Read the model definition and answer for the solid it produces. Units are mm, in the model's axes. Face numbers are marked on the shaded views. A direction names the side the tool comes from. Coordinates: 2 decimals unless noted, no trailing zeros. Loops run counter-clockwise (first coordinate to the right, second up) from the corner with the lowest first, then second, coordinate; pieces in that order, holes last. Notation, with made-up numbers: (23.25, -1.75) -> (40.25, -1.75) arc R37 cw to (40.25, 37.25) -> close; hole circle Ø6 at (21.25, -16.75). An arc over 180 degrees is marked (long way). Answer as a JSON object with one key per item and string values. Group by question number.
Q1. The part is cut by section D-D on y = 0. State how many separate pieces and enclosed holes the cut face has, and give its area (3 significant figures).
Q2. Each of these flat-tipped pins is pushed along its axis until it touches: P1, Ø2.5, axis at x = -7.2, y = 0, coming from the +Z side; P2, Ø3.5, axis at x = 0, y = -7.2, coming from the -Z side; P3, Ø8, axis at x = -5, z = -9, coming from the -Y side; P4, Ø4.5, axis at x = -1, y = 1, coming from the -Z side. Where does it stop, or does it pass through?
Q3. Determine the mould class of the marked faces 1, 2 and 3 for opening direction X: released by +X, released by -X, zero draft, split by the parting line, or undercut.
Q4. Straight lines are drawn through the part: line 1 along Y through (x, z) = (0, -0.7) (3 decimals); line 2 along Z through (x, y) = (4.75, -0.75); line 3 along Z through (x, y) = (5.5, 4.75). For each, find the intervals that lie inside material, in ascending order. Write a range as [from, to].
Q5. The part is cut by section A-A on y = 7.2. Write down the section's boundary in (x, z) (3 decimals), and give its area (3 significant figures).
Q6. The part is cut by section B-B on z = -1.5. Write down the section's boundary in (x, y) (3 decimals).
Q7. For the marked faces 4 and 5, determine the directions among +Z, -Z, +X, -X, +Y, -Y from which every point of the face is accessible in a straight line to the end or side of a thin tool.
from build123d import *

# Parameters (mm, degrees)
SKETCH_1_R               = 5
EXTRUDE_1_DEPTH          = 19.4
SKETCH_2_R               = 9.3
EXTRUDE_2_DEPTH          = 2.5
EXTRUDE_START            = 14.1
SKETCH_3_R               = 5
EXTRUDE_3_DEPTH          = 14.1
SKETCH_5_W               = 0.3
SKETCH_5_H               = 1.1
SKETCH_6_W               = 0.3
SKETCH_6_H               = 1.1
HOLE_WIZARD_M2_5_2_D     = 2.05
HOLE_WIZARD_M2_5_2_DEPTH = 7.25
HOLE_WIZARD_M2_5_2_TIP   = 0.591784026
SKETCH_12_R              = 2
CUT_EXTRUDE_1_DEPTH      = 28


with BuildPart() as part:
    # 草图1 → 凸台-拉伸1 (new body)
    with BuildSketch(Plane.XY):
        Circle(SKETCH_1_R)
    extrude(amount=EXTRUDE_1_DEPTH)

    # 草图2 → 凸台-拉伸2 (add)
    with BuildSketch(Plane(origin=(0, 0, 0), x_dir=(-1, 0, 0), z_dir=(0, 0, -1))):
        Circle(SKETCH_2_R)
    extrude(amount=EXTRUDE_2_DEPTH)

    # 草图3 → 凸台-拉伸3 (add)
    with BuildSketch(Plane(origin=(0, 0, -2.5), x_dir=(-1, 0, 0), z_dir=(0, 0, -1)).offset(EXTRUDE_START)):
        with Locations(Location((0, 0, 0), (0, 0, 180))):
            Circle(SKETCH_3_R)
    extrude(amount=-EXTRUDE_3_DEPTH)

    # 草图5 → 切除-旋转3 (revolve, cut)
    with BuildSketch(Plane(origin=(0, 0, 0), x_dir=(1, 0, 0), z_dir=(0, 1, 0)), mode=Mode.PRIVATE) as cut_revolve_3_sk:
        with Locations((4.85, 14.15)):
            Rectangle(SKETCH_5_W, SKETCH_5_H)
    revolve(cut_revolve_3_sk.sketch.rotate(Axis((0, 0, -16.6), (0, 0, 1)), 180), axis=Axis((0, 0, -16.6), (0, 0, 1)), mode=Mode.SUBTRACT)

    # 草图6 → 切除-旋转4 (revolve, cut)
    with BuildSketch(Plane(origin=(0, 0, 0), x_dir=(1, 0, 0), z_dir=(0, 1, 0))):
        with Locations((4.85, -16.95)):
            Rectangle(SKETCH_6_W, SKETCH_6_H)
    revolve(axis=Axis((0, 0, 19.4), (0, 0, -1)), mode=Mode.SUBTRACT)

    # M2.5 螺纹孔2
    with Locations(Plane(origin=(0, 7.2, -2.5), x_dir=(-1, 0, 0), z_dir=(0, 0, -1))):
        with Locations((0, 0), (7.2, -7.2), (-7.2, -7.2), (0, -14.4)):
            Hole(HOLE_WIZARD_M2_5_2_D / 2, depth=HOLE_WIZARD_M2_5_2_DEPTH)
            with Locations((0, 0, -(HOLE_WIZARD_M2_5_2_DEPTH + HOLE_WIZARD_M2_5_2_TIP / 2))):  # 120° drill point
                Cone(0, HOLE_WIZARD_M2_5_2_D / 2, HOLE_WIZARD_M2_5_2_TIP, mode=Mode.SUBTRACT)

    # 草图12 → 切除-拉伸1 (cut)
    with BuildSketch(Plane(origin=(0, 0, -16.6), x_dir=(-1, 0, 0), z_dir=(0, 0, -1))):
        Circle(SKETCH_12_R)
    extrude(amount=-CUT_EXTRUDE_1_DEPTH, mode=Mode.SUBTRACT)


solid = part.part
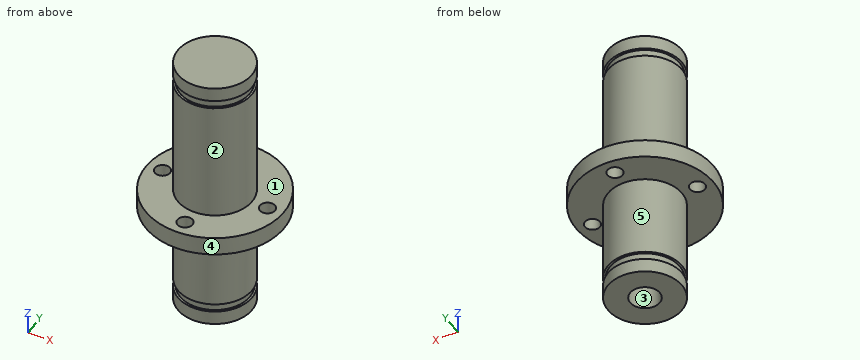
Final values:
{
 "1": {"separate pieces": "3", "enclosed holes": "0", "area": "258 mm2"},
 "2": {"P1": "stops at z = 0", "P2": "stops at z = -2.5", "P3": "stops at y = -4.9", "P4": "stops at z = -16.6"},
 "3": {"face 1": "zero draft", "face 2": "split by the parting line", "face 3": "undercut"},
 "4": {"line 1": "y = [-9.3, -8.225], [-6.175, -2], [2, 6.175], [8.225, 9.3]", "line 2": "z = [-16.6, -14.7], [-13.6, 16.4], [17.5, 19.4]", "line 3": "z = [-2.5, 0]"},
 "5": {"outline": "(-5.886, -2.5) -> (-1.025, -2.5) -> (-1.025, 0) -> (-5.886, 0) -> close; (1.025, -2.5) -> (5.886, -2.5) -> (5.886, 0) -> (1.025, 0) -> close", "area": "24.3 mm2"},
 "6": {"outline": "circle Ø18.6 at (0, 0); hole circle Ø2.05 at (-7.2, 0); hole circle Ø4 at (0, 0); hole circle Ø2.05 at (0, -7.2); hole circle Ø2.05 at (0, 7.2); hole circle Ø2.05 at (7.2, 0)"},
 "7": {"face 4": "+Z, -Z", "face 5": "-Z"}
}
